from build123d import *

# Parameters (mm, degrees)
F1_DEPTH = 101.6
F3_DEPTH = 25.4


with BuildPart() as f1:
    # F0 (on Front) → F1 (new body)
    with BuildSketch(Plane.XZ):
        Polygon((-35.885991, 6.716738), (-35.885991, -18.683262), (27.614009, -18.683262), (27.614009, 57.516738), (-10.485991, 57.516738), (-10.485991, 6.716738), align=None)
    extrude(amount=F1_DEPTH)

    # F2 (on Right) → F3 (cut)
    with BuildSketch(Plane.YZ):
        Polygon((-17.54909, 18.968504), (-17.54909, 57.19075), (-68.607166, 57.475988), (-68.607166, 18.968504), align=None)
    extrude(amount=-F3_DEPTH, mode=Mode.SUBTRACT)


solid = f1.part
Work out the finished part from the listing and answer in its coordinate system (mm). A direction names the side the tool comes from. Give positions to 0.01 mm unless a question says otherwise; leave off trailing zeros. Loops run counter-clockwise (first coordinate to the right, second up) from the corner with the lowest first, then second, coordinate; pieces in that order, holes last. Notation, with made-up numbers: (68.5, 37) -> (113.5, 37) arc R33 cw to (113.5, 72) -> close; hole circle Ø5 at (61.5, 19). An arc over 180 degrees is marked (long way). Use a Markdown table: item, result. Add a question column.
1) The part is cut by section C-C, the plane x = -25.5. Determine the outline of the cut face in (y, z), plus the area to 3 significant figures.
2) The part is cut by section B-B, the plane y = -25. Determine the outline of the cut face in (x, z), plus the area to 3 significant figures.
3) The part is cut by section A-A, the plane z = 36.5. Determine the outline of the cut face in (x, y), plus the area to 3 significant figures.
4) For a pull along Z with two mould halves and no side action, classify faces 1 (the flat face through (-5, -17.549, 38)), 2 (the flat face through (-35.886, -50, -6)), 3 (the flat face through (-23, -50, 6.717)) as +Z half, -Z half, draft (parallel to the pull), parting line (faces both ways), or undercut.
5) The part is cut by section D-D, the plane y = -70. Determine the outline of the cut face in (x, z), plus the area to 3 significant figures.
6) Each of these flat-tipped pins is pushed along its axis until it touches: P1, Ø1.5, axis at y = -22.5, z = 7, coming from the -X side; P2, Ø1.5, axis at y = -54, z = 49.5, coming from the -X side. Where does it stop, or does it pass through?
7) Which of the six approach directions +Z, -Z, +X, -X, +Y, -Y give full straight-line access (tool end or side, diameter ignored) to faces 4 (the flat face through (-10.486, -50, 16)), 5 (the flat face through (2, -101.6, 11)), 6 (the flat face through (-5, -68.607, 38))?
8) Consider line 1 along Y through (x, z) = (-7, 45); line 2 along X through (y, z) = (-52, 42); line 3 along X through (y, z) = (-48.5, 10.5). Determine where each line is inside the solid, lowest interval first.
Reported:
| question | item | result |
|---|---|---|
| 1 | outline | (-101.6, -18.68) -> (0, -18.68) -> (0, 6.72) -> (-101.6, 6.72) -> close |
| 1 | area | 2,580 mm^2 |
| 2 | outline | (-35.89, -18.68) -> (27.61, -18.68) -> (27.61, 57.52) -> (-10.49, 57.52) -> (-10.49, 57.23) -> (0, 57.23) -> (0, 18.97) -> (-10.49, 18.97) -> (-10.49, 6.72) -> (-35.89, 6.72) -> close |
| 2 | area | 3,150 mm^2 |
| 3 | outline | (-10.49, -101.6) -> (27.61, -101.6) -> (27.61, 0) -> (-10.49, 0) -> (-10.49, -17.55) -> (0, -17.55) -> (0, -68.61) -> (-10.49, -68.61) -> close |
| 3 | area | 3,340 mm^2 |
| 4 | face 1 | undercut |
| 4 | face 2 | draft |
| 4 | face 3 | +Z half |
| 5 | outline | (-35.89, -18.68) -> (27.61, -18.68) -> (27.61, 57.52) -> (-10.49, 57.52) -> (-10.49, 6.72) -> (-35.89, 6.72) -> close |
| 5 | area | 3,550 mm^2 |
| 6 | P1 | stops at x = -35.89 |
| 6 | P2 | stops at x = 0 |
| 7 | face 4 | +Z, -X, +Y, -Y |
| 7 | face 5 | +Z, -Z, +X, -X, -Y |
| 7 | face 6 | -X |
| 8 | line 1 | y = -101.6 to -68.61, -17.55 to 0 |
| 8 | line 2 | x = 0 to 27.61 |
| 8 | line 3 | x = -10.49 to 27.61 |
